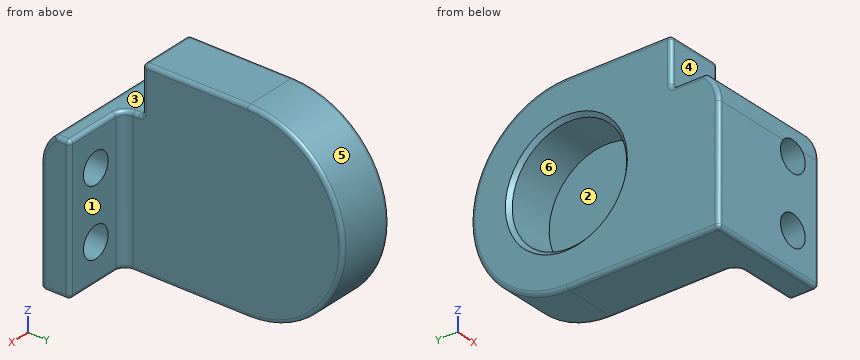
from build123d import *

# Parameters (mm, degrees)
SKETCH_1_R          = 3
EXTRUDE_1_DEPTH     = 3
SKETCH_2_W          = 3.5
SKETCH_2_H          = 10
SKETCH_2_R          = 0.8
EXTRUDE_2_DEPTH     = 1.5
SKETCH_5_W          = 6.5
SKETCH_5_H          = 2.5
CUT_EXTRUDE_1_DEPTH = 2.5
CUT_EXTRUDE_2_REACH = 13.456
FILLET_1_R          = 0.5
FILLET_2_R          = 0.2
CHAMFER_1_SIZE      = 0.2
SKETCH_3_R          = 3.977941141
EXTRUDE_3_DEPTH     = 0.4


with BuildPart() as part:
    # 草图1 → 凸台-拉伸1 (new body)
    with BuildSketch(Plane(origin=(0, 0, 0), x_dir=(0, 0, -1), z_dir=(1, 0, 0))):
        with BuildLine():
            Line((-5, 0), (-5, -8))
            Line((-5, -8), (5, -8))
            Line((5, -8), (5, 0))
            ThreePointArc((5, 0), (0, 5), (-5, 0))
        make_face()
        Circle(SKETCH_1_R, mode=Mode.SUBTRACT)
    extrude(amount=EXTRUDE_1_DEPTH)

    # 草图2 → 凸台-拉伸2 (add)
    with BuildSketch(Plane.XZ.offset(8)):
        with Locations((4.75, 0)):
            Rectangle(SKETCH_2_W, SKETCH_2_H)
        with Locations(Location((4.8, -3, 0), (0, 0, 270))):
            Circle(SKETCH_2_R, mode=Mode.SUBTRACT)
        with Locations(Location((4.8, 0.5, 0), (0, 0, 270))):
            Circle(SKETCH_2_R, mode=Mode.SUBTRACT)
    extrude(amount=-EXTRUDE_2_DEPTH)

    # 草图5 → 切除-拉伸1 (cut)
    with BuildSketch(Plane.XZ.offset(8)):
        with Locations((3.25, 3.75)):
            Rectangle(SKETCH_5_W, SKETCH_5_H)
    extrude(amount=-CUT_EXTRUDE_1_DEPTH, mode=Mode.SUBTRACT)

    # 草图6 → 切除-拉伸2 (cut, up to next)
    with BuildSketch(Plane.ZY, mode=Mode.PRIVATE) as cut_extrude_2_sk1:
        with BuildLine():
            Line((2.897366596, -6), (3.27705392, -6))
            Line((3.27705392, -6), (3.27705392, -8.325127743))
            Line((3.27705392, -8.325127743), (1, -8.325127743))
            Line((1, -8.325127743), (1, -8))
            ThreePointArc((1, -8), (2.378404875, -7.407669683), (2.897366596, -6))
        make_face()
    cut_extrude_2_tool1 = extrude(cut_extrude_2_sk1.sketch, amount=-CUT_EXTRUDE_2_REACH, mode=Mode.PRIVATE) & part.part
    add(cut_extrude_2_tool1.solids().sort_by_distance((0, -7.575754, 2.569334))[0], mode=Mode.SUBTRACT)

    # 圆角1
    fillet_1_edges = [part.edges().sort_by_distance(p)[0] for p in [
        (3, -6.5, -1.25),
    ]]
    fillet(fillet_1_edges, radius=FILLET_1_R)

    # 圆角2
    fillet_2_edges = [part.edges().sort_by_distance(p)[0] for p in [
        (6.5, -6.5, -1.25),
        (6.5, -7.25, -5),
        (6.5, -8, -2),
        (3, 5, 0),
        (0, -5.5, 3.75),
        (0, -6.383095189, 2.5),
        (1.5, -5.5, 5),
        (6.5, -6.883095189, 2.5),
        (1.5, -5.5, 2.5),
        (3, -5.5, 3.75),
        (0, -4, -5),
        (0, -2.75, 5),
        (0, 5, 0),
        (0, -8, -2),
        (3.25, -7.266190379, 2.5),
        (6.5, -7.806716397, 1.834936608),
        (0, -7.806716397, 1.834936608),
        (3, -5.75, 2.5),
        (3, -3, -5),
        (5, -6.5, 2.5),
        (3, -2.75, 5),
        (5, -6.5, -5),
        (3.146446609, -6.353553391, -5),
        (3.146446609, -6.353553391, 2.5),
        (3.25, -8, -5),
    ]]
    fillet(fillet_2_edges, radius=FILLET_2_R)

    # 倒角1
    chamfer_1_edges = [part.edges().sort_by_distance(p)[0] for p in [
        (0, 0, 3),
        (3, 0, 3),
    ]]
    chamfer(chamfer_1_edges, length=CHAMFER_1_SIZE)

    # 草图3 → 凸台-拉伸3 (add)
    with BuildSketch(Plane(origin=(3, 0, 0), x_dir=(0, 0, -1), z_dir=(1, 0, 0))):
        Circle(SKETCH_3_R)
    extrude(amount=-EXTRUDE_3_DEPTH)


solid = part.part
Model file for the job. Use its own axes, mm. Face numbers are marked on the shaded views. A direction names the side the tool comes from. Give positions to 0.01 mm unless a question says otherwise; leave off trailing zeros. Write each loop counter-clockwise with the first axis right and the second up, starting at its lowest first coordinate (ties: lowest second). Pieces come first, ordered by that corner, then holes. Notation, with made-up numbers: (78.5, -14) -> (84.5, -14) arc R14 cw to (84.5, 5) -> close; hole circle Ø3 at (54.5, 58). An arc over 180 degrees is marked (long way). Write item = value, one per line.
(1) Mould opens along Z. For the marked faces 4, 5 and 6 say: released by +Z, released by -Z, zero draft, split by the parting line, or undercut.
Determined:
face_4 = zero draft
face_5 = split by the parting line
face_6 = undercut
(2) Slice it at A-A, the plane x = 1. Give the cut face in (y, z), then the cut area to 3 significant figures.
Determined:
outline = (-8, -4.8) arc R0.2 ccw to (-7.8, -5) -> (0, -5) arc R5 ccw to (0, 5) -> (-5.3, 5) arc R0.2 ccw to (-5.5, 4.8) -> (-5.5, 2.7) arc R0.2 cw to (-5.7, 2.5) -> (-7.2, 2.5) arc R0.2 ccw to (-7.32, 2.45) arc R1.9 ccw to (-8, 1) -> close; hole circle Ø6 at (0, 0)
area = 84.4 mm2
(3) Slice it at C-C, the plane z = 0. Give the cut face in (x, y).
Determined:
outline = (0, -7.8) arc R0.2 ccw to (0.2, -8) -> (4.18, -8) -> (4.18, -6.5) -> (3.5, -6.5) arc R0.5 cw to (3, -6) -> (3, 4.8) arc R0.2 ccw to (2.8, 5) -> (0.2, 5) arc R0.2 ccw to (0, 4.8) -> (0, 3.2) -> (0.2, 3) -> (2.6, 3) -> (2.6, -3) -> (0.2, -3) -> (0, -3.2) -> close; (5.42, -8) -> (6.3, -8) arc R0.2 ccw to (6.5, -7.8) -> (6.5, -6.7) arc R0.2 ccw to (6.3, -6.5) -> (5.42, -6.5) -> close
(4) Flat gauge pins, fed straight in: P1, Ø3, axis at x = 5, z = -2, coming from the +Y side; P2, Ø0.6, axis at x = 1, z = 3.5, coming from the -Y side; P3, Ø3, axis at x = 1.5, y = 2.5, coming from the +Z side. Where does each tip first touch, or does it go through?
Determined:
P1 = -6.5
P2 = -5.5
P3 = 4.9
(5) Slice it at D-D, the plane x = 3.75. Give the cut face in (y, z), then the cut area to 3 significant figures.
Determined:
outline = (-8, -4.8) arc R0.2 ccw to (-7.8, -5) -> (-6.7, -5) arc R0.2 ccw to (-6.5, -4.8) -> (-6.5, 2.3) arc R0.2 ccw to (-6.7, 2.5) -> (-7.2, 2.5) arc R0.2 ccw to (-7.32, 2.45) arc R1.9 ccw to (-8, 1) -> close
area = 10.9 mm2
(6) Probe line 1 along Y through (x, z) = (1.15, 0); line 2 along Z through (x, y) = (0.9, 0); line 3 along X through (y, z) = (-7.1, 0.5). List the from-to ranges inside material, lowest first.
Determined:
line_1 = -8 to -3, 3 to 5
line_2 = -5 to -3, 3 to 5
line_3 = 0 to 4, 5.6 to 6.5
(7) Slice it at B-B, the plane y = -7. Give the cut face in (x, z).
Determined:
outline = (0, -4.8) arc R0.2 ccw to (0.2, -5) -> (6.3, -5) arc R0.2 ccw to (6.5, -4.8) -> (6.5, 2.3) arc R0.2 ccw to (6.3, 2.5) -> (0.2, 2.5) arc R0.2 ccw to (0, 2.3) -> close; hole circle Ø1.6 at (4.8, -3); hole circle Ø1.6 at (4.8, 0.5)
(8) Tool access for the marked faces 1, 2 and 3: list every direction of +Z, -Z, +X, -X, +Y, -Y with a clear straight run to the whole face (end or side of a thin tool).
Determined:
face_1 = +Z, -Z, +X, +Y
face_2 = -X
face_3 = +Z, +X, -X, -Y
